```python
from build123d import *

# Parameters (mm, degrees)
EXTRUDE_1_DEPTH            = 50
HOLE_WIZARD_M51_AT_2_COUNT = 2
HOLE_WIZARD_M51_AT_2_PITCH = 30
HOLE_WIZARD_M51_AT_3_COUNT = 2
HOLE_WIZARD_M51_AT_3_PITCH = 58
HOLE_WIZARD_M51_AT_4_COUNT = 2
HOLE_WIZARD_M51_AT_4_PITCH = 88


with BuildPart() as part:
    # Эскиз1 → Бобышка-Вытянуть1 (new body, symmetric)
    with BuildSketch(Plane.XY):
        Polygon((3, 0), (-3, 0), (-3, -0.9), (-5.1, -0.9), (-5.1, -1.9), (-3, -5), (3, -5), (5.1, -1.9), (5.1, -0.9), (3, -0.9), align=None)
    extrude(amount=EXTRUDE_1_DEPTH, both=True)

    # Эскиз4 → Отверстие обработанное метчиком M51 (revolve, cut)
    with BuildSketch(Plane(origin=(0, 0, -44), x_dir=(0, 0, 1), z_dir=(1, 0, 0))):
        Polygon((0, 0), (0, 5), (2.525, 5), (2.1, 4.575), (2.1, 0.425), (2.525, 0), align=None)
    hole_wizard_m51 = revolve(axis=Axis((0, 6.35, -44), (0, -1, 0)), mode=Mode.SUBTRACT)

    # Отверстие обработанное метчиком M51 at 2: Отверстие обработанное метчиком M51 ×2
    with Locations(*[(0, 0, i * HOLE_WIZARD_M51_AT_2_PITCH) for i in range(1, HOLE_WIZARD_M51_AT_2_COUNT)]):
        add(hole_wizard_m51, mode=Mode.SUBTRACT)

    # Отверстие обработанное метчиком M51 at 3: Отверстие обработанное метчиком M51 ×2
    with Locations(*[(0, 0, i * HOLE_WIZARD_M51_AT_3_PITCH) for i in range(1, HOLE_WIZARD_M51_AT_3_COUNT)]):
        add(hole_wizard_m51, mode=Mode.SUBTRACT)

    # Отверстие обработанное метчиком M51 at 4: Отверстие обработанное метчиком M51 ×2
    with Locations(*[(0, 0, i * HOLE_WIZARD_M51_AT_4_PITCH) for i in range(1, HOLE_WIZARD_M51_AT_4_COUNT)]):
        add(hole_wizard_m51, mode=Mode.SUBTRACT)


solid = part.part
```
Here's how the part is built. I have some questions about the finished solid (model axes, mm). A direction names the side the tool comes from. Coordinates: 2 decimals unless noted, no trailing zeros. Order: outer loops, then holes, each group sorted by start corner. A loop starts at its lowest first (then second) coordinate and runs counter-clockwise, first axis right, second up. Notation, with made-up numbers: (69.5, 73) - (91.5, 73) arc R18 ccw to (91.5, 101) - close; hole circle Ø7 at (-40, 7.5). An arc over 180 degrees is marked (long way). One line per question, with ' | ' between items.
(1) Suppose I cut it at B-B on y = -2.65. List the corners of the cut face in (x, z) for me, and give its area (3 significant figures).
Report:
outline: (-4.59, -50) - (4.59, -50) - (4.59, 50) - (-4.59, 50) - close; hole circle Ø4.2 at (0, -44); hole circle Ø4.2 at (0, -14); hole circle Ø4.2 at (0, 14); hole circle Ø4.2 at (0, 44) | area: 863 mm2
(2) Suppose I cut it at A-A on z = -14. List the corners of the cut face in (x, y) for me (3 decimals).
Report:
outline: (-5.1, -1.9) - (-3, -5) - (-2.525, -5) - (-2.1, -4.575) - (-2.1, -0.425) - (-2.525, 0) - (-3, 0) - (-3, -0.9) - (-5.1, -0.9) - close; (2.1, -4.575) - (2.525, -5) - (3, -5) - (5.1, -1.9) - (5.1, -0.9) - (3, -0.9) - (3, 0) - (2.525, 0) - (2.1, -0.425) - close
(3) If I drill on L1, parallel to Z at x = 0, y = -1.9; L2, parallel to Z at x = -2, y = -0.3 (3 decimals); L3, parallel to X at y = -1.35, z = -14, over which ranges is the centre line in solid material (lowest first)?
Report:
L1: z = -50 to -46.1, -41.9 to -16.1, -11.9 to 11.9, 16.1 to 41.9, 46.1 to 50 | L2: z = -50 to -44.975, -43.025 to -14.975, -13.025 to 13.025, 14.975 to 43.025, 44.975 to 50 | L3: x = -5.1 to -2.1, 2.1 to 5.1
(4) Will these pins go through, and if not, where does the flat tip stop? pin 1 (1 mm diameter, centred on x = -4, z = 21, fed in from +Y); pin 2 (3.5 mm diameter, centred on x = 0, z = 44, fed in from +Y); pin 3 (2 mm diameter, centred on y = -4, z = 32.5, fed in from -X).
Report:
pin 1: stops at y = -0.9 | pin 2: passes through | pin 3: stops at x = -4.35
(5) Suppose I cut it at C-C on x = 0. State how many separate pieces and enclosed holes the cut face has, and give its area (3 significant figures).
Report:
separate pieces: 5 | enclosed holes: 0 | area: 415 mm2
(6) For faces 1 (the flat face through (4, -0.9, 1)), 2 (the flat face through (-4, -0.9, 1)), 3 (the cylindrical face through (-0.09, -2.47, 11.9)), which set-ups out of +Z, -Z, +X, -X, +Y, -Y let a thin tool reach every point of the face, with its end or its side?
Report:
face 1: +Z, -Z, +X, +Y | face 2: +Z, -Z, -X, +Y | face 3: +Y, -Y
(7) Suppose I cut it at D-D on x = -4.25. List the corners of the cut face in (y, z) for me, and give its area (3 significant figures).
Report:
outline: (-3.15, -50) - (-0.9, -50) - (-0.9, 50) - (-3.15, 50) - close | area: 225 mm2
